Design review of the part built by this model. Coordinates are the model's own, in mm. Coordinates: 2 decimals unless noted, no trailing zeros. Loops run counter-clockwise (first coordinate to the right, second up) from the corner with the lowest first, then second, coordinate; pieces in that order, holes last. Notation, with made-up numbers: M -21.75,44 L 33.25,44 A26 ccw 33.25,73 Z; hole C 50.25,65 d5. An arc over 180 degrees is marked long. Put each result on its own line as item: value. Start each with the question number.
(1) Take a section at B-B, the plane x = 38.1. Give the boundary of the cut face in (y, z), then the cut area to 3 significant figures.
(2) For probe 1 along X at (y, z) = (2, 44.45); probe 2 along X at (y, z) = (3.25, -50.8); probe 3 along Z at (x, y) = (15, 5.75), list the stretches that pass through material, from the lowest coordinate up. Write a range as [from, to].
(3) Take a section at C-C, the plane z = 44.45. Give the boundary of the cut face in (x, y).
(4) Take a section at A-A, the plane y = 3.5. Count the separate pieces of the cut face and the enclosed holes in it, then the cut area to 3 significant figures.
(5) Clearance check with flat-ended pins moving along their axes: pin 1 (7.5 mm diameter, centred on x = 38.1, z = 44.45, fed in from +Y); pin 2 (8 mm diameter, centred on x = -7, z = 45, fed in from -Y); pin 3 (3 mm diameter, centred on x = -39, y = 2, fed in from -Z); pin 4 (3 mm diameter, centred on y = 4, z = -4.5, fed in from +X). State where each tip first meets the part, or that it passes through.
(6) Take a section at D-D, the plane x = -1.5. Give the boundary of the cut face in (y, z), then the cut area to 3 significant figures.
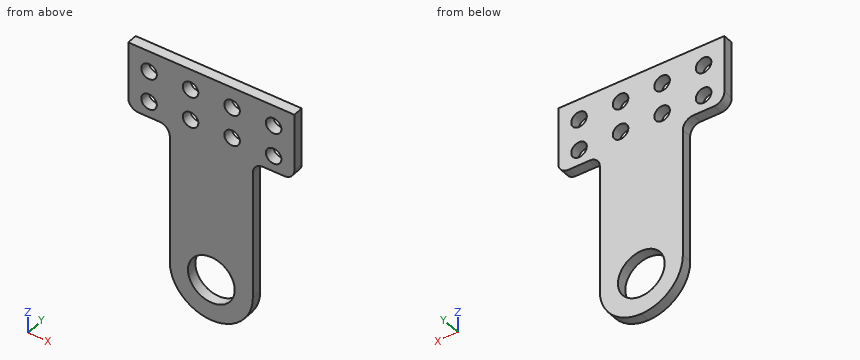
```python
from build123d import *

# Parameters (mm, degrees)
SKETCH1_W            = 25.4
SKETCH1_H            = 41.493412961
SKETCH1_W_2          = 50.8
SKETCH1_H_2          = 110.906587039
BOSS_EXTRUDE1_DEPTH  = 6.35
SKETCH2_R            = 14.3002
CUT_EXTRUDE1_DEPTH   = 6.35
SKETCH3_R            = 4.7625
CUT_EXTRUDE2_DEPTH   = 6.35
LPATTERN1_COUNT      = 4
LPATTERN1_PITCH      = 25.4
LPATTERN1_COUNT_DIR2 = 2
LPATTERN1_PITCH_DIR2 = 19.05
FILLET1_R            = 6.35
FILLET2_R            = 25.4


with BuildPart() as part:
    # Sketch1 → Boss-Extrude1 (new body)
    with BuildSketch(Plane(origin=(0, 0, 0), x_dir=(1, 0, 0), z_dir=(0, 1, 0))):
        with Locations((-38.1, -55.45329352)):
            Rectangle(SKETCH1_W, SKETCH1_H)
        with Locations((0, -55.45329352)):
            Rectangle(SKETCH1_W_2, SKETCH1_H)
        with Locations((0, 20.746706481)):
            Rectangle(SKETCH1_W_2, SKETCH1_H_2)
        with Locations((38.1, -55.45329352)):
            Rectangle(SKETCH1_W, SKETCH1_H)
    extrude(amount=BOSS_EXTRUDE1_DEPTH)

    # Sketch2 → Cut-Extrude1 (cut)
    with BuildSketch(Plane(origin=(0, 6.35, 0), x_dir=(1, 0, 0), z_dir=(0, 1, 0))):
        with Locations(Location((0, 50.8, 0), (0, 0, 270))):
            Circle(SKETCH2_R)
    extrude(amount=-CUT_EXTRUDE1_DEPTH, mode=Mode.SUBTRACT)

    # Sketch3 → Cut-Extrude2 (cut)
    with BuildSketch(Plane(origin=(0, 6.35, 0), x_dir=(1, 0, 0), z_dir=(0, 1, 0))):
        with Locations(Location((-38.1, -63.5, 0), (0, 0, 270))):
            Circle(SKETCH3_R)
    cut_extrude2 = extrude(amount=-CUT_EXTRUDE2_DEPTH, mode=Mode.SUBTRACT)

    # LPattern1: Cut-Extrude2 4 × 2
    with Locations(*[(i * LPATTERN1_PITCH, 0, -j * LPATTERN1_PITCH_DIR2) for i in range(LPATTERN1_COUNT) for j in range(LPATTERN1_COUNT_DIR2) if (i, j) != (0, 0)]):
        add(cut_extrude2, mode=Mode.SUBTRACT)

    # Fillet1
    fillet1_edges = [part.edges().sort_by_distance(p)[0] for p in [
        (-50.8, 3.175, 34.706587039),
        (-25.4, 3.175, 34.706587039),
        (25.4, 3.175, 34.706587039),
        (50.8, 3.175, 34.706587039),
    ]]
    fillet(fillet1_edges, radius=FILLET1_R)

    # Fillet2
    fillet2_edges = [part.edges().sort_by_distance(p)[0] for p in [
        (25.4, 3.175, -76.2),
        (-25.4, 3.175, -76.2),
    ]]
    fillet(fillet2_edges, radius=FILLET2_R - 0.0001)  # a hair under: the kernel refuses the full size


solid = part.part
```
Computed values:
1. outline: M 0,34.71 L 6.35,34.71 L 6.35,39.69 L 0,39.69 Z; M 0,49.21 L 6.35,49.21 L 6.35,58.74 L 0,58.74 Z; M 0,68.26 L 6.35,68.26 L 6.35,76.2 L 0,76.2 Z
1. area: 143 mm^2
2. probe 1: x = [-50.8, -42.86], [-33.34, -17.46], [-7.94, 7.94], [17.46, 33.34], [42.86, 50.8]
2. probe 2: x = [-25.4, -14.3], [14.3, 25.4]
2. probe 3: z = [-71.3, 40.28], [48.62, 59.33], [67.67, 76.2]
3. outline: M -50.8,0 L -42.86,0 L -42.86,6.35 L -50.8,6.35 Z; M -33.34,0 L -17.46,0 L -17.46,6.35 L -33.34,6.35 Z; M -7.94,0 L 7.94,0 L 7.94,6.35 L -7.94,6.35 Z; M 17.46,0 L 33.34,0 L 33.34,6.35 L 17.46,6.35 Z; M 42.86,0 L 50.8,0 L 50.8,6.35 L 42.86,6.35 Z
4. separate pieces: 1
4. enclosed holes: 9
4. area: 8,360 mm^2
5. pin 1: passes through
5. pin 2: stops at y = 0
5. pin 3: stops at z = 34.71
5. pin 4: stops at x = 25.4
6. outline: M 0,-76.16 L 6.35,-76.16 L 6.35,-65.02 L 0,-65.02 Z; M 0,-36.58 L 6.35,-36.58 L 6.35,76.2 L 0,76.2 Z
6. area: 787 mm^2
